For this review, take the finished solid that the model builds, in its own axes (mm). Face numbers are marked on the shaded views. Round coordinates to 2 decimals unless told otherwise and drop trailing zeros. Loops run counter-clockwise (first coordinate to the right, second up) from the corner with the lowest first, then second, coordinate; pieces in that order, holes last.
1. Consider section B-B on y = 1. State the section outline as (x, z) points, then the cut area to 3 significant figures.
2. Consider section D-D on x = -34. State the section outline as (y, z) points, then the cut area to 3 significant figures.
3. Consider section A-A on x = 52. State the section outline as (y, z) points.
4. Consider section C-C on x = -5. State the section outline as (y, z) points, then the cut area to 3 significant figures.
5. Draft analysis for pull direction X (two halves, no side actions). For the marked faces 1, 2, 3 and 4, state which applies: released by +X, released by -X, zero draft, split by the parting line, or undercut.
6. To check wall thickness, follow line 1 along X through (y, z) = (2.4, 0.5); line 2 along X through (y, z) = (1.6, -1.5); line 3 along X through (y, z) = (-1.8, 0.5). State the ranges of each line that lie inside material, in increasing order.
7. Clearance check with flat-ended pins moving along their axes: pin 1 Ø10 at (x, z) = (-16.5, -5.5) entering from +Y; pin 2 Ø3 at (x, z) = (-52, 0.5) entering from -Y; pin 3 Ø2 at (x, y) = (-15, 6.5) entering from -Z. State where each tip first meets the part, or that it passes through.
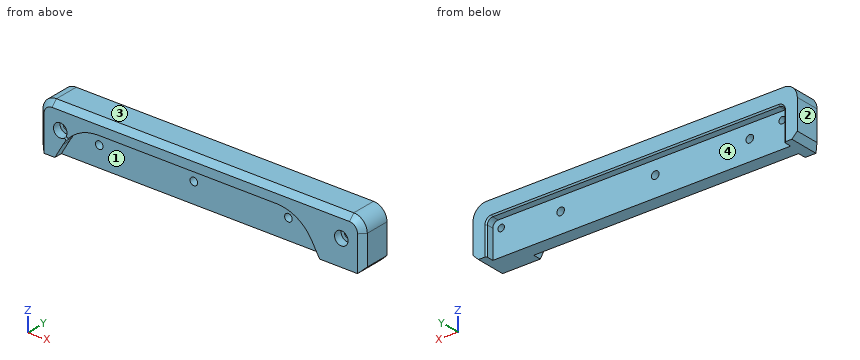
from build123d import *

# Parameters (mm, degrees)
SKETCH_1_W      = 120
SKETCH_1_H      = 18
SKETCH_1_R      = 1.4
SKETCH_1_R_2    = 1.2
EXTRUDE_1_DEPTH = 5
EXTRUDE_2_DEPTH = 3
SKETCH_3_R      = 2.5
EXTRUDE_3_DEPTH = 3
FILLET_1_R      = 5
CHAMFER_1_SIZE  = 0.5
CHAMFER_2_SIZE  = 2
CHAMFER_3_SIZE  = 2


with BuildPart() as part:
    # Sketch 1 → Extrude 1 (new body)
    with BuildSketch(Plane(origin=(0, 0, 0), x_dir=(1, 0, 0), z_dir=(0, 1, 0))):
        Rectangle(SKETCH_1_W, SKETCH_1_H)
        with Locations(Location((30, 1.5, 0), (0, 0, 270))):
            Circle(SKETCH_1_R, mode=Mode.SUBTRACT)
        with Locations(Location((-5, 1.5, 0), (0, 0, 270))):
            Circle(SKETCH_1_R, mode=Mode.SUBTRACT)
        with Locations(Location((-40, 1.5, 0), (0, 0, 270))):
            Circle(SKETCH_1_R, mode=Mode.SUBTRACT)
        with Locations(Location((52, -0.5, 0), (0, 0, 270))):
            Circle(SKETCH_1_R_2, mode=Mode.SUBTRACT)
        with Locations(Location((-52, -0.5, 0), (0, 0, 270))):
            Circle(SKETCH_1_R_2, mode=Mode.SUBTRACT)
    extrude(amount=EXTRUDE_1_DEPTH)

    # Sketch 2 → Extrude 2 (add)
    with BuildSketch(Plane(origin=(0, 5, 0), x_dir=(1, 0, 0), z_dir=(0, 1, 0))):
        with BuildLine():
            Line((-55.1, 9), (-55.1, -1.5))
            ThreePointArc((-55.1, -1.5), (-54.514213562, -2.914213562), (-53.1, -3.5))
            Line((-53.1, -3.5), (53.1, -3.5))
            ThreePointArc((53.1, -3.5), (54.514213562, -2.914213562), (55.1, -1.5))
            Line((55.1, -1.5), (55.1, 9))
            Line((55.1, 9), (60, 9))
            Line((60, 9), (60, -9))
            Line((60, -9), (-60, -9))
            Line((-60, -9), (-60, 9))
            Line((-60, 9), (-55.1, 9))
        make_face()
    extrude(amount=EXTRUDE_2_DEPTH)

    # Sketch 3 → Extrude 3 (add)
    with BuildSketch(Plane.XZ):
        with BuildLine():
            Line((-50.990381057, -3.8), (-53.992602457, -9))
            Line((-53.992602457, -9), (-60, -9))
            Line((-60, -9), (-60, 9))
            Line((-60, 9), (60, 9))
            Line((60, 9), (60, -9))
            Line((60, -9), (43.992602457, -9))
            Line((43.992602457, -9), (40.990381057, -3.8))
            ThreePointArc((40.990381057, -3.8), (35.5, 1.690381057), (28, 3.7))
            Line((28, 3.7), (-38, 3.7))
            ThreePointArc((-38, 3.7), (-43.896602634, 2.492392011), (-48.843767341, -0.935989683))
            ThreePointArc((-48.843767341, -0.935989683), (-49.473949116, -1.012171842), (-49.671021877, -0.408768893))
            ThreePointArc((-49.671021877, -0.408768893), (-53.911569658, 2.11118014), (-50.710028515, -1.641488634))
            ThreePointArc((-50.710028515, -1.641488634), (-50.081970455, -1.733553091), (-50.050355695, -2.367535187))
            ThreePointArc((-50.050355695, -2.367535187), (-50.540837816, -3.070334948), (-50.990381057, -3.8))
        make_face()
        with Locations(Location((52, 0.5, 0), (0, 0, 270))):
            Circle(SKETCH_3_R, mode=Mode.SUBTRACT)
    extrude(amount=EXTRUDE_3_DEPTH)

    # Fillet 1
    fillet_1_edges = [part.edges().sort_by_distance(p)[0] for p in [
        (60, 2.5, 9),
        (-60, 2.5, 9),
    ]]
    fillet(fillet_1_edges, radius=FILLET_1_R)

    # Chamfer 1
    chamfer_1_edges = [part.edges().sort_by_distance(p)[0] for p in [
        (55.1, 8, -3.75),
        (54.514213562, 8, 2.914213562),
        (0, 8, 3.5),
        (-54.514213562, 8, 2.914213562),
        (-55.1, 8, -3.75),
    ]]
    chamfer(chamfer_1_edges, length=CHAMFER_1_SIZE)

    # Chamfer 2
    chamfer_2_edges = [part.edges().sort_by_distance(p)[0] for p in [
        (-60, 2.5, -9),
        (60, 2.5, -9),
    ]]
    chamfer(chamfer_2_edges, length=CHAMFER_2_SIZE)

    # Chamfer 3
    chamfer_3_edges = [part.edges().sort_by_distance(p)[0] for p in [
        (60, -3, -1.5),
        (-60, -3, -1.5),
        (58.535533906, -3, 7.535533906),
        (-58.535533906, -3, 7.535533906),
        (0, -3, 9),
    ]]
    chamfer(chamfer_3_edges, length=CHAMFER_3_SIZE)


solid = part.part
Resolved:
1. outline: (-60, -7) - (-58, -9) - (58, -9) - (60, -7) - (60, 4) arc R5 ccw to (55, 9) - (-55, 9) arc R5 ccw to (-60, 4) - close; hole circle Ø2.4 at (-52, 0.5); hole circle Ø2.8 at (-40, -1.5); hole circle Ø2.8 at (-5, -1.5); hole circle Ø2.8 at (30, -1.5); hole circle Ø2.4 at (52, 0.5)
1. area: 2,120 mm2
2. outline: (-3, 3.7) - (0, 3.7) - (0, -9) - (5, -9) - (5, 3.5) - (7.5, 3.5) - (8, 4) - (8, 9) - (-1, 9) - (-3, 7) - close
2. area: 120 mm2
3. outline: (-3, -9) - (5, -9) - (5, -0.7) - (0, -0.7) - (0, -2) - (-3, -2) - close; (-3, 3) - (0, 3) - (0, 1.7) - (5, 1.7) - (5, 3.5) - (7.5, 3.5) - (8, 4) - (8, 9) - (-1, 9) - (-3, 7) - close
4. outline: (-3, 3.7) - (0, 3.7) - (0, -0.1) - (5, -0.1) - (5, 3.5) - (7.5, 3.5) - (8, 4) - (8, 9) - (-1, 9) - (-3, 7) - close; (0, -9) - (5, -9) - (5, -2.9) - (0, -2.9) - close
4. area: 106 mm2
5. face 1: undercut
5. face 2: released by -X
5. face 3: zero draft
5. face 4: undercut
6. line 1: x = -60 to -53.2, -50.8 to 50.8, 53.2 to 60
6. line 2: x = -60 to -41.4, -38.6 to -6.4, -3.6 to 28.6, 31.4 to 60
6. line 3: x = -59.2 to -54.5, -49.5 to -47.26, 37.26 to 49.5, 54.5 to 59.2
7. pin 1: stops at y = 5
7. pin 2: stops at y = 0
7. pin 3: stops at z = 3.5
